Part print with two shaded views. Sizes in mm from the minimum x, y, z corner. A direction names the side the tool comes from. Coordinates: 2 decimals unless noted, no trailing zeros. Loops run counter-clockwise (first coordinate to the right, second up) from the corner with the lowest first, then second, coordinate; pieces in that order, holes last. Notation, with made-up numbers: (3, -29.75) -> (49, -29.75) arc R24 cw to (49, -11.75) -> close; hole circle Ø9 at (65.5, 64). An arc over 180 degrees is marked (long way). Write each question's results on one line, items separated by ' | '.
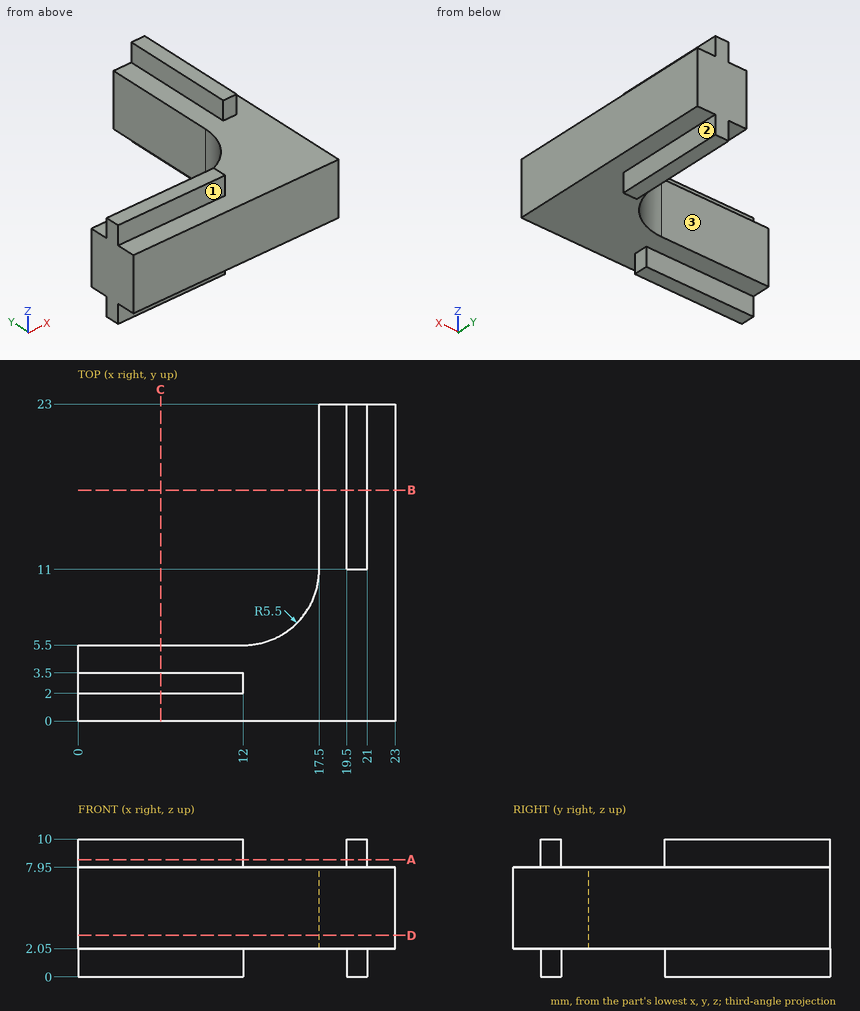
Q1. Cut at B-B on y = 16.75. Write the cut outline in (x, z), and give its area (3 significant figures).
Results are:
outline: (17.5, 2.05) -> (19.5, 2.05) -> (19.5, 0) -> (21, 0) -> (21, 2.05) -> (23, 2.05) -> (23, 7.95) -> (21, 7.95) -> (21, 10) -> (19.5, 10) -> (19.5, 7.95) -> (17.5, 7.95) -> close | area: 38.6 mm^2
Q2. Cut at D-D on z = 3. Write the cut outline in (x, y), and give its area (3 significant figures).
Results are:
outline: (0, 0) -> (23, 0) -> (23, 23) -> (17.5, 23) -> (17.5, 11) arc R5.5 cw to (12, 5.5) -> (0, 5.5) -> close | area: 229 mm^2
Q3. Cut at A-A on z = 8.5. Write the cut outline in (x, y), and give its area (3 significant figures).
Results are:
outline: (0, 2) -> (12, 2) -> (12, 3.5) -> (0, 3.5) -> close; (19.5, 11) -> (21, 11) -> (21, 23) -> (19.5, 23) -> close | area: 36.0 mm^2
Q4. Which spindle directions (+Z, -Z, +X, -X, +Y, -Y) get a long thin tool onto all of the face, cutting with end or side? Do the marked faces 1, 2 and 3. Say none if no direction does.
Results are:
face 1: +Z, +X, -X, -Y | face 2: -Z, +X, +Y, -Y | face 3: +Z, -Z, -X, +Y
Q5. Wall check: L1, parallel to X at y = 18, z = 9.25; L2, parallel to Y at x = 7.25, z = 4.25; L3, parallel to X at y = 16.5, z = 6. Give the ranges that are in metal, low to high. Write a range as from..to.
Results are:
L1: 19.5..21 | L2: 0..5.5 | L3: 17.5..23
Q6. Cut at C-C on x = 6. Write the cut outline in (y, z).
Results are:
outline: (0, 2.05) -> (2, 2.05) -> (2, 0) -> (3.5, 0) -> (3.5, 2.05) -> (5.5, 2.05) -> (5.5, 7.95) -> (3.5, 7.95) -> (3.5, 10) -> (2, 10) -> (2, 7.95) -> (0, 7.95) -> close
Q7. Drop flat-ended pins along their axis: pin 1 (1.6 mm diameter, centred on x = 7, z = 9, fed in from +Y); pin 2 (6 mm diameter, centred on x = 16, y = 5, fed in from +Z); pin 3 (0.6 mm diameter, centred on x = 6.5, z = 9, fed in from -Y). Give the stop position or say it passes through.
Results are:
pin 1: y = 3.5 | pin 2: z = 7.95 | pin 3: y = 2
